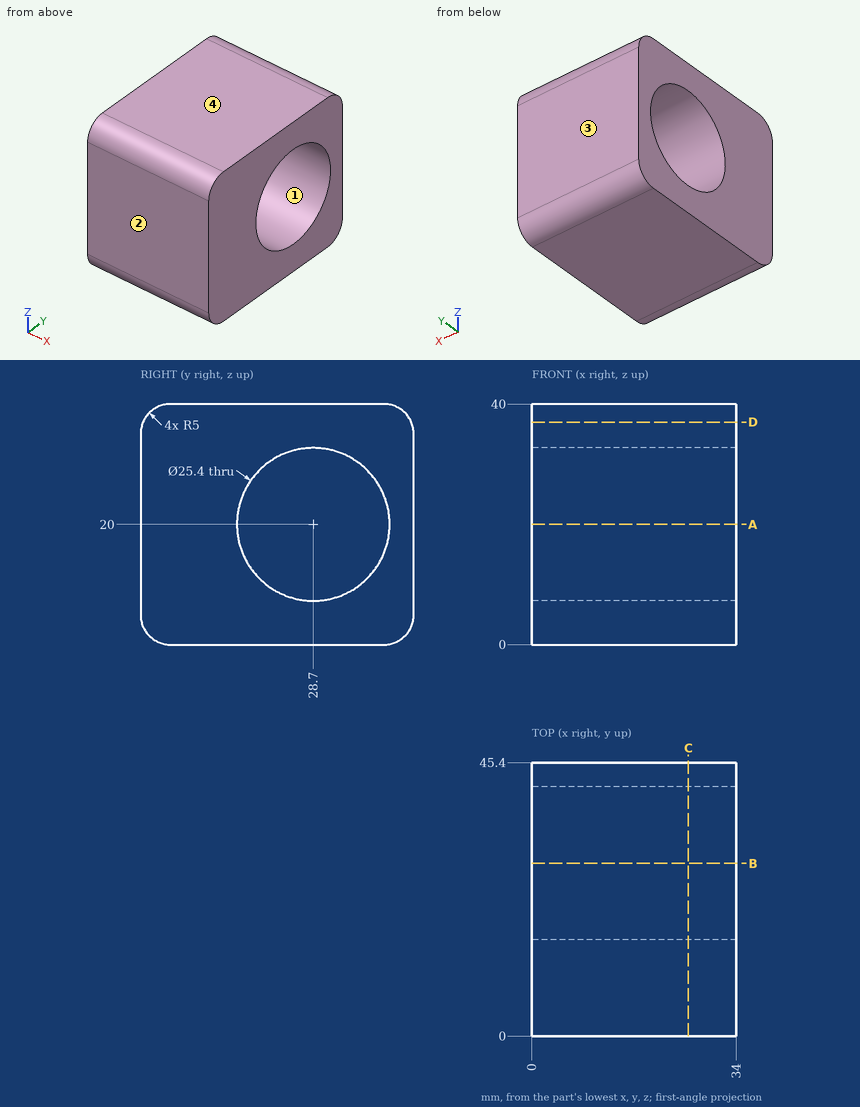
Here's the drawing with two shaded views (mm, measured from the low corner). I have some questions. Round coordinates to 2 decimals unless told otherwise and drop trailing zeros. Write each loop counter-clockwise with the first axis right and the second up, starting at its lowest first coordinate (ties: lowest second). Pieces come first, ordered by that corner, then holes. Notation, with made-up numbers: M 46.25,78.25 L 89.25,78.25 A16 cw 89.25,90.25 Z; hole C -26.75,27 d7. An arc over 180 degrees is marked long. Answer in a Markdown table with one row per item. Add a question column.
Q1. Imagine slicing it at A-A (z = 20). Please give me the cut outline in (x, y), then the cut area to 3 significant figures.
Q2. If we mould it in two halves opening along Y, with no side actions, what happens to the marked faces 1, 2, 3 and 4? For each: +Y half, -Y half, draft (parallel to the pull), parting line (faces both ways), or undercut.
Q3. Imagine slicing it at D-D (z = 37). Please give me the cut outline in (x, y).
Q4. Imagine slicing it at B-B (y = 28.7). Please give me the cut outline in (x, z).
Q5. Imagine slicing it at C-C (x = 26). Please give me the cut outline in (y, z).
Q6. If I drill on line 1 (Y direction, x = 22.5, z = 20); line 2 (Z direction, x = 14.5, y = 17.5); line 3 (Z direction, x = 25, y = 28), over which ranges is the centre line in solid material (lowest first)? Write a range as from..to.
Values:
| question | item | result |
|---|---|---|
| 1 | outline | M 0,0 L 34,0 L 34,16 L 0,16 Z; M 0,41.4 L 34,41.4 L 34,45.4 L 0,45.4 Z |
| 1 | area | 680 mm^2 |
| 2 | face 1 | undercut |
| 2 | face 2 | -Y half |
| 2 | face 3 | +Y half |
| 2 | face 4 | draft |
| 3 | outline | M 0,0.42 L 34,0.42 L 34,44.98 L 0,44.98 Z |
| 4 | outline | M 0,0 L 34,0 L 34,7.3 L 0,7.3 Z; M 0,32.7 L 34,32.7 L 34,40 L 0,40 Z |
| 5 | outline | M 0,5 A5 ccw 5,0 L 40.4,0 A5 ccw 45.4,5 L 45.4,35 A5 ccw 40.4,40 L 5,40 A5 ccw 0,35 Z; hole C 28.7,20 d25.4 |
| 6 | line 1 | 0..16, 41.4..45.4 |
| 6 | line 2 | 0..14.01, 25.99..40 |
| 6 | line 3 | 0..7.32, 32.68..40 |
